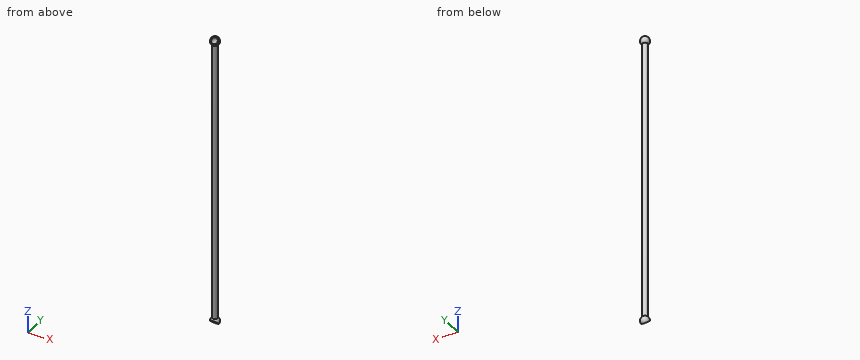
```python
from build123d import *

# Parameters (mm, degrees)
SKETCH1_R                = 4
BOSS_EXTRUDE1_DEPTH      = 214.080811
BOSS_EXTRUDE1_DEPTH_BACK = 214.080811
CUT_EXTRUDE1_START       = -10.192388155
SKETCH5_W                = 20
SKETCH5_H                = 5
CUT_EXTRUDE1_DEPTH       = 318.544568669


with BuildPart() as part:
    # Sketch1 → Boss-Extrude1 (new body, two sides)
    with BuildSketch(Plane.XY) as boss_extrude1_sk:
        Circle(SKETCH1_R)
    extrude(amount=BOSS_EXTRUDE1_DEPTH)
    extrude(boss_extrude1_sk.sketch, amount=-BOSS_EXTRUDE1_DEPTH_BACK)

    # Sketch3 → Revolve1 (revolve)
    with BuildSketch(Plane(origin=(0, 0, 0), x_dir=(0, 0, -1), z_dir=(1, 0, 0))):
        with BuildLine():
            Line((-220.580811107, 0), (-207.580811107, 0))
            ThreePointArc((-207.580811107, 0), (-214.080811107, 6.5), (-220.580811107, 0))
        make_face()
    revolve1 = revolve(axis=Axis((0, 0, 220.580811107), (0, 0, -1)))

    # Sketch5 → Cut-Extrude1 (cut)
    with BuildSketch(Plane(origin=(0, 107.040405554, 107.040405554), x_dir=(1, 0, 0), z_dir=(0, -0.707106781, -0.707106781)).offset(CUT_EXTRUDE1_START)):
        with Locations((0, 155.877993256)):
            Rectangle(SKETCH5_W, SKETCH5_H)
    cut_extrude1 = extrude(amount=CUT_EXTRUDE1_DEPTH, mode=Mode.SUBTRACT)

    # Sketch6 → Cut-Revolve1 (revolve, cut)
    with BuildSketch(Plane(origin=(0, 0, 0), x_dir=(1, 0, 0), z_dir=(0, 1, 0))):
        with BuildLine():
            Line((0, -209.080811107), (0, -219.080811107))
            ThreePointArc((0, -219.080811107), (5, -214.080811107), (0, -209.080811107))
        make_face()
    cut_revolve1 = revolve(axis=Axis((0, 0, 209.080811107), (0, 0, 1)), mode=Mode.SUBTRACT)

    # Mirror2: Revolve1, Cut-Extrude1, Cut-Revolve1 across plane
    add(revolve1.mirror(Plane.XY))
    add(cut_extrude1.mirror(Plane.XY), mode=Mode.SUBTRACT)
    add(cut_revolve1.mirror(Plane.XY), mode=Mode.SUBTRACT)


solid = part.part
```
Model file for the job. Use its own axes, mm. Coordinates: 2 decimals unless noted, no trailing zeros. Write each loop counter-clockwise with the first axis right and the second up, starting at its lowest first coordinate (ties: lowest second). Pieces come first, ordered by that corner, then holes. Notation, with made-up numbers: (33.5, -21) - (51.5, -21) arc R22 ccw to (51.5, -8) - close; hole circle Ø11 at (26.25, 66). An arc over 180 degrees is marked (long way). Use a Markdown table: item, result. Add a question column.
Item 1: Band-saw the part on B-B, the plane x = 0. Write the cut outline in (y, z).
Item 2: Drop flat-ended pins along their axis: pin 1 (6 mm diameter, centred on y = -4, z = 134.5, fed in from -X); pin 2 (1.5 mm diameter, centred on x = -3.5, z = -77.5, fed in from -Y); pin 3 (5 mm diameter, centred on y = -2.5, z = 35.5, fed in from -X). Give the stop position or say it passes through.
Item 3: Drill centre lines: line 1 along Y through (x, z) = (-0.5, -26.5); line 2 along Z through (x, y) = (3.25, 1); line 3 along Z through (x, y) = (-4.5, 0.5). Where is each one in solid material? Low to high.
Item 4: Band-saw the part on A-A, the plane z = 4.5. Write the cut outline in (x, y), and give its area (3 significant figures).
Item 5: Band-saw the part on C-C, the plane y = 0. Write the cut outline in (x, z), and give its area (3 significant figures).
A:
| question | item | result |
|---|---|---|
| 1 | outline | (-5.79, -211.12) - (-4.65, -212.25) arc R5 cw (long way) to (1.83, -218.74) - (2.96, -219.87) arc R6.5 ccw to (4, -208.96) - (4, 208.96) arc R6.5 ccw to (2.96, 219.87) - (1.83, 218.74) arc R5 cw (long way) to (-4.65, 212.25) - (-5.79, 211.12) arc R6.5 ccw to (-4, 208.96) - (-4, -208.96) arc R6.5 ccw to start |
| 2 | pin 1 | stops at x = -3.87 |
| 2 | pin 2 | stops at y = -2.9 |
| 2 | pin 3 | stops at x = -4 |
| 3 | line 1 | y = -3.97 to 3.97 |
| 3 | line 2 | z = -217.91 to -217.75, -210.42 to 210.42, 217.75 to 217.91 |
| 3 | line 3 | z = -217.41 to -216.2, -211.96 to -209.42, 209.42 to 211.96, 216.2 to 217.41 |
| 4 | outline | circle Ø8 at (0, 0) |
| 4 | area | 50.3 mm² |
| 5 | outline | (-5.85, -216.91) - (-4.12, -216.91) arc R5 cw (long way) to (4.12, -216.91) - (5.85, -216.91) arc R6.5 ccw to (4, -208.96) - (4, 208.96) arc R6.5 ccw to (5.85, 216.91) - (4.12, 216.91) arc R5 cw (long way) to (-4.12, 216.91) - (-5.85, 216.91) arc R6.5 ccw to (-4, 208.96) - (-4, -208.96) arc R6.5 ccw to start |
| 5 | area | 3,400 mm² |
